The listing builds one solid part. Answer for the finished solid, in the listing's coordinates (mm). A direction names the side the tool comes from. Coordinates: 2 decimals unless noted, no trailing zeros. Order: outer loops, then holes, each group sorted by start corner. A loop starts at its lowest first (then second) coordinate and runs counter-clockwise, first axis right, second up. Notation, with made-up numbers: (-31, 46.5) - (0, 46.5) arc R23 cw to (0, 81.5) - close; hole circle Ø6 at (-33.5, -19). An arc over 180 degrees is marked (long way). Use a Markdown table: item, result. Add a question column.
Item 1: The part is cut by section C-C, the plane z = 16.5. Give the vertices of the cut face in (x, y), then the cut area to 3 significant figures.
Item 2: Find the intervals of material crossed by line 1 along X through (y, z) = (92.95, 30); line 2 along Y through (x, z) = (201.4, 35); line 3 along Y through (x, z) = (156, 21.5), in increasing order.
Item 3: For faces 1 (the flat face through (101, 90, 30)), 2 (the cylindrical face through (27.284, 92.028, 29.479)), 3 (the flat face through (202, 25, 30)), determine the directions among +Z, -Z, +X, -X, +Y, -Y from which every point of the face is accessible in a straight line to the end or side of a thin tool.
Item 4: A flat-ended cylindrical pin translates along its axis: P1, Ø6, axis at y = 49.5, z = 6.5, coming from the -X side. Find the tip coordinate at first contact, or state that the pin passes through.
Item 5: The part is cut by section B-B, the plane x = 96.5. Give the vertices of the cut face in (y, z), then the cut area to 3 significant figures.
Item 6: The mould has two halves that part along Y. Classify faces 4 (the flat face through (202, 45, 20)), 5 (the flat face through (103, -4, 30)), 6 (the cylindrical face through (2.85, -1.97, 3.01)): released by +Y, released by -Y, zero draft, split by the parting line, or undercut.
Item 7: The part is cut by section A-A, the plane y = 21.5. Give the vertices of the cut face in (x, z).
Item 8: The part is cut by section D-D, the plane z = 30. State how many separate pieces and enclosed holes the cut face has, then the cut area to 3 significant figures.
from build123d import *

# Parameters (mm, degrees)
EKSTR_ZYON_NCE1_DEPTH = 60
RADYUS1_R             = 10
KES_EKSTR_ZYON1_REACH = 236.137
IZIM2_R               = 4
IZIM2_R_2             = 2
KES_EKSTR_ZYON2_REACH = 234.491
IZIM3_R               = 2
IZIM3_W               = 20
IZIM3_H               = 40


with BuildPart() as part:
    # izim1 → Ekstr_zyon-_nce1 (new body)
    with BuildSketch(Plane.XY):
        Polygon((0, 0), (200, 0), (200, 90), (0, 90), (0, 94), (204, 94), (204, -4), (0, -4), align=None)
    extrude(amount=EKSTR_ZYON_NCE1_DEPTH)

    # Radyus1
    radyus1_edges = [part.edges().sort_by_distance(p)[0] for p in [
        (0, -2, 60),
        (0, 92, 60),
        (0, -2, 0),
        (0, 92, 0),
    ]]
    fillet(radyus1_edges, radius=RADYUS1_R)

    # izim2 → Kes-Ekstr_zyon1 (cut, up to next)
    with BuildSketch(Plane(origin=(0, 94, 0), x_dir=(1, 0, 0), z_dir=(0, 1, 0)), mode=Mode.PRIVATE) as kes_ekstr_zyon1_sk1:
        with Locations(Location((23.318126504, -30, 0), (0, 0, 270))):
            Circle(IZIM2_R)
    kes_ekstr_zyon1_tool1 = extrude(kes_ekstr_zyon1_sk1.sketch, amount=-KES_EKSTR_ZYON1_REACH, mode=Mode.PRIVATE) & part.part
    # izim2 → Kes-Ekstr_zyon1 (cut, up to next)
    with BuildSketch(Plane(origin=(0, 94, 0), x_dir=(1, 0, 0), z_dir=(0, 1, 0)), mode=Mode.PRIVATE) as kes_ekstr_zyon1_sk2:
        with Locations(Location((23.318126504, -22, 0), (0, 0, 270))):
            Circle(IZIM2_R_2)
    kes_ekstr_zyon1_tool2 = extrude(kes_ekstr_zyon1_sk2.sketch, amount=-KES_EKSTR_ZYON1_REACH, mode=Mode.PRIVATE) & part.part
    # izim2 → Kes-Ekstr_zyon1 (cut, up to next)
    with BuildSketch(Plane(origin=(0, 94, 0), x_dir=(1, 0, 0), z_dir=(0, 1, 0)), mode=Mode.PRIVATE) as kes_ekstr_zyon1_sk3:
        with Locations(Location((23.318126504, -38, 0), (0, 0, 270))):
            Circle(IZIM2_R_2)
    kes_ekstr_zyon1_tool3 = extrude(kes_ekstr_zyon1_sk3.sketch, amount=-KES_EKSTR_ZYON1_REACH, mode=Mode.PRIVATE) & part.part
    # izim2 → Kes-Ekstr_zyon1 (cut, up to next)
    with BuildSketch(Plane(origin=(0, 94, 0), x_dir=(1, 0, 0), z_dir=(0, 1, 0)), mode=Mode.PRIVATE) as kes_ekstr_zyon1_sk4:
        with Locations(Location((31.318126504, -30, 0), (0, 0, 270))):
            Circle(IZIM2_R_2)
    kes_ekstr_zyon1_tool4 = extrude(kes_ekstr_zyon1_sk4.sketch, amount=-KES_EKSTR_ZYON1_REACH, mode=Mode.PRIVATE) & part.part
    # izim2 → Kes-Ekstr_zyon1 (cut, up to next)
    with BuildSketch(Plane(origin=(0, 94, 0), x_dir=(1, 0, 0), z_dir=(0, 1, 0)), mode=Mode.PRIVATE) as kes_ekstr_zyon1_sk5:
        with Locations(Location((15.318126504, -30, 0), (0, 0, 270))):
            Circle(IZIM2_R_2)
    kes_ekstr_zyon1_tool5 = extrude(kes_ekstr_zyon1_sk5.sketch, amount=-KES_EKSTR_ZYON1_REACH, mode=Mode.PRIVATE) & part.part
    kes_ekstr_zyon1_1 = kes_ekstr_zyon1_tool1.solids().sort_by_distance((23.318127, 94, 30))[0]
    add(kes_ekstr_zyon1_1, mode=Mode.SUBTRACT)
    kes_ekstr_zyon1_2 = kes_ekstr_zyon1_tool2.solids().sort_by_distance((23.318127, 94, 22))[0]
    add(kes_ekstr_zyon1_2, mode=Mode.SUBTRACT)
    kes_ekstr_zyon1_3 = kes_ekstr_zyon1_tool3.solids().sort_by_distance((23.318127, 94, 38))[0]
    add(kes_ekstr_zyon1_3, mode=Mode.SUBTRACT)
    kes_ekstr_zyon1_4 = kes_ekstr_zyon1_tool4.solids().sort_by_distance((31.318127, 94, 30))[0]
    add(kes_ekstr_zyon1_4, mode=Mode.SUBTRACT)
    kes_ekstr_zyon1_5 = kes_ekstr_zyon1_tool5.solids().sort_by_distance((15.318127, 94, 30))[0]
    add(kes_ekstr_zyon1_5, mode=Mode.SUBTRACT)
    kes_ekstr_zyon1 = kes_ekstr_zyon1_1 + kes_ekstr_zyon1_2 + kes_ekstr_zyon1_3 + kes_ekstr_zyon1_4 + kes_ekstr_zyon1_5  # Kes-Ekstr_zyon1 as one shape, for the pattern or mirror that repeats it

    # Aynalama1: Kes-Ekstr_zyon1 across plane
    add(kes_ekstr_zyon1.mirror(Plane.ZX.offset(45)), mode=Mode.SUBTRACT)

    # izim3 → Kes-Ekstr_zyon2 (cut, up to next)
    with BuildSketch(Plane(origin=(204, 0, 0), x_dir=(0, 0, -1), z_dir=(1, 0, 0)), mode=Mode.PRIVATE) as kes_ekstr_zyon2_sk1:
        with Locations((-25, 68.5)):
            Circle(IZIM3_R)
    kes_ekstr_zyon2_tool1 = extrude(kes_ekstr_zyon2_sk1.sketch, amount=-KES_EKSTR_ZYON2_REACH, mode=Mode.PRIVATE) & part.part
    # izim3 → Kes-Ekstr_zyon2 (cut, up to next)
    with BuildSketch(Plane(origin=(204, 0, 0), x_dir=(0, 0, -1), z_dir=(1, 0, 0)), mode=Mode.PRIVATE) as kes_ekstr_zyon2_sk2:
        with Locations(Location((-35, 68.5, 0), (0, 0, 180))):
            Circle(IZIM3_R)
    kes_ekstr_zyon2_tool2 = extrude(kes_ekstr_zyon2_sk2.sketch, amount=-KES_EKSTR_ZYON2_REACH, mode=Mode.PRIVATE) & part.part
    # izim3 → Kes-Ekstr_zyon2 (cut, up to next)
    with BuildSketch(Plane(origin=(204, 0, 0), x_dir=(0, 0, -1), z_dir=(1, 0, 0)), mode=Mode.PRIVATE) as kes_ekstr_zyon2_sk3:
        with Locations(Location((-25, 21.5, 0), (0, 0, 180))):
            Circle(IZIM3_R)
    kes_ekstr_zyon2_tool3 = extrude(kes_ekstr_zyon2_sk3.sketch, amount=-KES_EKSTR_ZYON2_REACH, mode=Mode.PRIVATE) & part.part
    # izim3 → Kes-Ekstr_zyon2 (cut, up to next)
    with BuildSketch(Plane(origin=(204, 0, 0), x_dir=(0, 0, -1), z_dir=(1, 0, 0)), mode=Mode.PRIVATE) as kes_ekstr_zyon2_sk4:
        with Locations((-35, 21.5)):
            Circle(IZIM3_R)
    kes_ekstr_zyon2_tool4 = extrude(kes_ekstr_zyon2_sk4.sketch, amount=-KES_EKSTR_ZYON2_REACH, mode=Mode.PRIVATE) & part.part
    # izim3 → Kes-Ekstr_zyon2 (cut, up to next)
    with BuildSketch(Plane(origin=(204, 0, 0), x_dir=(0, 0, -1), z_dir=(1, 0, 0)), mode=Mode.PRIVATE) as kes_ekstr_zyon2_sk5:
        with Locations((-30, 45)):
            Rectangle(IZIM3_W, IZIM3_H)
    kes_ekstr_zyon2_tool5 = extrude(kes_ekstr_zyon2_sk5.sketch, amount=-KES_EKSTR_ZYON2_REACH, mode=Mode.PRIVATE) & part.part
    add(kes_ekstr_zyon2_tool1.solids().sort_by_distance((204, 68.5, 25))[0], mode=Mode.SUBTRACT)
    add(kes_ekstr_zyon2_tool2.solids().sort_by_distance((204, 68.5, 35))[0], mode=Mode.SUBTRACT)
    add(kes_ekstr_zyon2_tool3.solids().sort_by_distance((204, 21.5, 25))[0], mode=Mode.SUBTRACT)
    add(kes_ekstr_zyon2_tool4.solids().sort_by_distance((204, 21.5, 35))[0], mode=Mode.SUBTRACT)
    add(kes_ekstr_zyon2_tool5.solids().sort_by_distance((204, 45, 30))[0], mode=Mode.SUBTRACT)


solid = part.part
Solution:
| question | item | result |
|---|---|---|
| 1 | outline | (0, -4) - (204, -4) - (204, 94) - (0, 94) - (0, 90) - (200, 90) - (200, 0) - (0, 0) - close |
| 1 | area | 1,990 mm2 |
| 2 | line 1 | x = 0 to 13.32, 17.32 to 19.32, 27.32 to 29.32, 33.32 to 204 |
| 2 | line 2 | y = -4 to 19.5, 23.5 to 25, 65 to 66.5, 70.5 to 94 |
| 2 | line 3 | y = -4 to 0, 90 to 94 |
| 3 | face 1 | +Z, -Z, -X |
| 3 | face 2 | +Y, -Y |
| 3 | face 3 | +X, -X |
| 4 | P1 | stops at x = 200 |
| 5 | outline | (-4, 0) - (0, 0) - (0, 60) - (-4, 60) - close; (90, 0) - (94, 0) - (94, 60) - (90, 60) - close |
| 5 | area | 480 mm2 |
| 6 | face 4 | undercut |
| 6 | face 5 | released by -Y |
| 6 | face 6 | zero draft |
| 7 | outline | (200, 0) - (204, 0) - (204, 23) - (200, 23) - close; (200, 27) - (204, 27) - (204, 33) - (200, 33) - close; (200, 37) - (204, 37) - (204, 60) - (200, 60) - close |
| 8 | separate pieces | 8 |
| 8 | enclosed holes | 0 |
| 8 | area | 1,700 mm2 |
